Autodesk Inventor part; units mm, degrees
ref_plane "YZ Plane" through (0, 0, 0) normal (1, 0, 0) x (0, 1, 0)
ref_plane "XZ Plane" through (0, 0, 0) normal (0, 1, 0) x (-1, 0, 0)
ref_plane "XY Plane" through (0, 0, 0) normal (0, 0, 1) x (1, 0, 0)
sketch "Skizze1" plane through (0, 0, 0) normal (0, 1, 0) x (-1, 0, 0)
  line L0 (6, 0) -> (3, -5.1962)
  line L1 (3, -5.1962) -> (-3, -5.1962)
  line L2 (-3, -5.1962) -> (-6, 0)
  line L3 (-6, 0) -> (-3, 5.1962)
  line L4 (-3, 5.1962) -> (3, 5.1962)
  line L5 (3, 5.1962) -> (6, 0)
  point P0 (0, 0)
  point P1 (0, 0)
  dimension "d5" = 12
extrude "Extrusion3" add sketch "Skizze1" along normal blind 3
sketch "Sketch4" plane through (0, 3, 0) normal (0, 1, 0) x (1, 0, 0)
  circle A0 centre (0, 0) radius 5
  dimension "d12" = 10
extrude "Extrusion4" add sketch "Sketch4" along normal blind 11.5
sketch "Sketch5" plane through (0, 14.5, 0) normal (0, 1, 0) x (1, 0, 0)
  circle A0 centre (0, 0) radius 5 construction
hole "Hole1" at (0, 14.5, 0) direction (0, -1, 0) diameter 8 depth 14.5
properties part number "überwurfmutter" material "Gold"
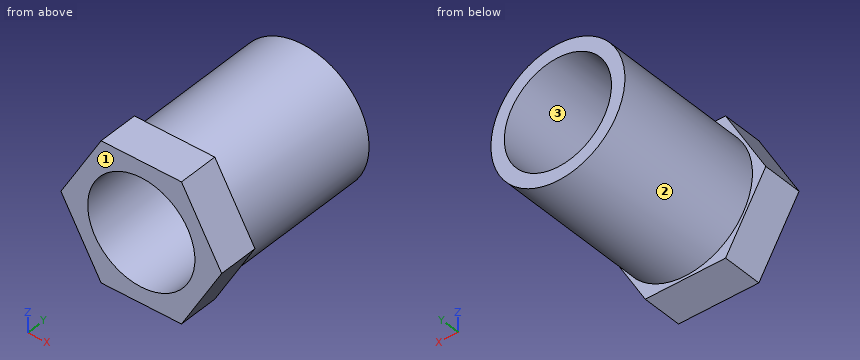
Build history of the part. All positions in model axes, mm. Face numbers are marked on the shaded views. Round coordinates to 2 decimals unless told otherwise and drop trailing zeros. Write each loop counter-clockwise with the first axis right and the second up, starting at its lowest first coordinate (ties: lowest second). Pieces come first, ordered by that corner, then holes.
1) Pin check, flat tips, straight feed: pin 1 (4 mm diameter, centred on x = 4, y = 10.5, fed in from -Z); pin 2 (1 mm diameter, centred on x = -4, y = 10, fed in from +Z); pin 3 (1 mm diameter, centred on y = 6, z = -2, fed in from +X). Stop position of each tip, or through.
2) Drill centre lines: probe 1 along Z at (x, y) = (0, 3.5); probe 2 along Y at (x, z) = (-5, 1.5). Where is each one in solid material? Low to high.
3) Mould opens along Z. For the marked faces 1, 2 and 3 say: +Z half, -Z half, draft (parallel to the pull), parting line (faces both ways), or undercut.
4) Band-saw the part on D-D, the plane z = -4.5. List the corners of the cut face in (x, y).
5) Band-saw the part on B-B, the plane z = -1.5. List the corners of the cut face in (x, y).
6) Band-saw the part on A-A, the plane x = 0. List the corners of the cut face in (y, z).
7) Band-saw the part on C-C, the plane y = 5.75. List the corners of the cut face in (x, z).
Ans:
1. pin 1: stops at z = -4.58
1. pin 2: stops at z = 3.57
1. pin 3: stops at x = 4.77
2. probe 1: z = -5 to -4, 4 to 5
2. probe 2: y = 0 to 3
3. face 1: draft
3. face 2: parting line
3. face 3: undercut
4. outline: (-3.4, 0) - (3.4, 0) - (3.4, 3) - (2.18, 3) - (2.18, 14.5) - (-2.18, 14.5) - (-2.18, 3) - (-3.4, 3) - close
5. outline: (-5.13, 0) - (-3.71, 0) - (-3.71, 14.5) - (-4.77, 14.5) - (-4.77, 3) - (-5.13, 3) - close; (3.71, 0) - (5.13, 0) - (5.13, 3) - (4.77, 3) - (4.77, 14.5) - (3.71, 14.5) - close
6. outline: (0, -5.2) - (3, -5.2) - (3, -5) - (14.5, -5) - (14.5, -4) - (0, -4) - close; (0, 4) - (14.5, 4) - (14.5, 5) - (3, 5) - (3, 5.2) - (0, 5.2) - close
7. outline: circle Ø10 at (0, 0); hole circle Ø8 at (0, 0)
